```python
from build123d import *

# Parameters (mm, degrees)
BOX_W        = 8
BOX_H        = 15
BOX_DEPTH    = 3
SKETCH_R     = 11
PAD_DEPTH    = 2
SKETCH001_R  = 9.5
PAD001_DEPTH = 15
SKETCH002_R  = 9.25
PAD002_DEPTH = 23
SKETCH003_R  = 8.5
POCKET_DEPTH = 2
SKETCH004_R  = 7.5
PAD003_DEPTH = 2


with BuildPart() as cubo:
    # Box → Box (new body)
    with BuildSketch(Plane(origin=(-4, 15, 8), x_dir=(1, 0, 0), z_dir=(0, 0, 1))):
        with Locations((4, 7.5)):
            Rectangle(BOX_W, BOX_H)
    extrude(amount=BOX_DEPTH)


with BuildPart() as fusion:
    # Sketch → Pad (new body)
    with BuildSketch(Plane.XZ):
        Circle(SKETCH_R)
    extrude(amount=PAD_DEPTH)

    # Sketch001 (on Face2 of Pad) → Pad001 (join)
    with BuildSketch(Plane(origin=(0, 0, 0), x_dir=(1, 0, 0), z_dir=(0, 1, 0))):
        Circle(SKETCH001_R)
    extrude(amount=PAD001_DEPTH)

    # Sketch002 (on Face5 of Pad001) → Pad002 (join)
    with BuildSketch(Plane(origin=(0, 15, 0), x_dir=(1, 0, 0), z_dir=(0, 1, 0))):
        Circle(SKETCH002_R)
    extrude(amount=PAD002_DEPTH)

    # Sketch003 (on Face3 of Pad002) → Pocket (cut)
    with BuildSketch(Plane.XZ.offset(2)):
        Circle(SKETCH003_R)
    extrude(amount=-POCKET_DEPTH, mode=Mode.SUBTRACT)

    # Sketch004 (on Face7 of Pocket) → Pad003 (join)
    with BuildSketch(Plane.XZ):
        Circle(SKETCH004_R)
    extrude(amount=PAD003_DEPTH)

    # Fusion: union Cubo
    add(cubo.part)


solid = fusion.part
```
The model under review builds one solid part; all positions refer to its coordinate system, in mm. A direction names the side the tool comes from. Round coordinates to 2 decimals unless told otherwise and drop trailing zeros. Write each loop counter-clockwise with the first axis right and the second up, starting at its lowest first coordinate (ties: lowest second). Pieces come first, ordered by that corner, then holes. Notation, with made-up numbers: M -26.75,-38 L 25.25,-38 A12 cw 25.25,-16 Z; hole C 10.25,24.5 d9. An arc over 180 degrees is marked long. Use CSV: the item, a comma, the result in double quotes. Start each with the question number.
(1) Tool access review of faces 1 (the face through (0, 0, -8)), 2 (the face through (4, 22, 10)), 3 (the face through (-1.2, 26.34, -9.17)), 4 (the face through (-10, 0, 0)), 5 (the face through (-4, 22, 10)): name each direction out of +Z, -Z, +X, -X, +Y, -Y from which nothing blocks a thin tool from reaching the whole face with its end or side.
(2) We need section A-A, the plane x = 0. State the section outline as (y, z) points.
(3) We need section C-C, the plane y = 24. State the section outline as (x, z) points.
(4) We need section D-D, the plane x = 5. State the section outline as (y, z) points.
(5) Clearance check with flat-ended pins moving along their axes: P1, Ø3, axis at x = 3, y = 13.5, coming from the -Z side; P2, Ø6, axis at y = 12, z = 4, coming from the +X side; P3, Ø4, axis at y = 33.5, z = 2.5, coming from the -X side. State where each tip first meets the part, or that it passes through.
(6) We need section B-B, the plane z = 0. State the section outline as (x, y) points, then the cut area to 4 significant figures.
(7) The part is to be moulded in two halves that separate along X. For faces 6 (the face through (4.57, -1.014, 7.167)), 7 (the face through (0, 30, 10)), 8 (the face through (-2.38, -0.99, -10.74)), 9 (the face through (-7.493, -0.986, 0.33)), say which applies: +X half, -X half, draft (parallel to the pull), parting line (faces both ways), or undercut.
(8) For line 1 along Z through (x, y) = (0, -1.4); line 2 along Y through (x, z) = (-3.75, 6.75); line 3 along Z through (x, y) = (0.25, 25.5), list the stretches that pass through material, from the lowest coordinate up.
Findings:
1,face 1,"-Y"
1,face 2,"+Z, +X, +Y"
1,face 3,"+Y"
1,face 4,"none"
1,face 5,"+Z, -X, +Y"
2,outline,"M -2,-11 L 0,-11 L 0,-9.5 L 15,-9.5 L 15,-9.25 L 38,-9.25 L 38,9.25 L 30,9.25 L 30,11 L 15,11 L 15,9.5 L 0,9.5 L 0,11 L -2,11 L -2,8.5 L 0,8.5 L 0,7.5 L -2,7.5 L -2,-7.5 L 0,-7.5 L 0,-8.5 L -2,-8.5 Z"
3,outline,"M -4,8.34 A9.25 ccw long 4,8.34 L 4,11 L -4,11 Z"
4,outline,"M -2,-9.8 L 0,-9.8 L 0,-8.08 L 15,-8.08 L 15,-7.78 L 38,-7.78 L 38,7.78 L 15,7.78 L 15,8.08 L 0,8.08 L 0,9.8 L -2,9.8 L -2,6.87 L 0,6.87 L 0,5.59 L -2,5.59 L -2,-5.59 L 0,-5.59 L 0,-6.87 L -2,-6.87 Z"
5,P1,"z = -9.38"
5,P2,"x = 9.45"
5,P3,"x = -9.24"
6,outline,"M -11,-2 L -8.5,-2 L -8.5,0 L -7.5,0 L -7.5,-2 L 7.5,-2 L 7.5,0 L 8.5,0 L 8.5,-2 L 11,-2 L 11,0 L 9.5,0 L 9.5,15 L 9.25,15 L 9.25,38 L -9.25,38 L -9.25,15 L -9.5,15 L -9.5,0 L -11,0 Z"
6,area,"750.5 mm^2"
7,face 6,"undercut"
7,face 7,"draft"
7,face 8,"parting line"
7,face 9,"undercut"
8,line 1,"-11 to -8.5, -7.5 to 7.5, 8.5 to 11"
8,line 2,"0 to 38"
8,line 3,"-9.25 to 11"
